```python
from build123d import *

# Parameters (mm, degrees)
PAD015_DEPTH        = 70.75
REVOLUTION002_ANGLE = 180
SKETCH027_R         = 1.375
POCKET008_DEPTH     = 17.751
SKETCH028_R         = 2.5
POCKET009_DEPTH     = 9.751
FILLET001_R         = 0.75


with BuildPart() as part:
    # Sketch025 → Pad015 (new body)
    with BuildSketch(Plane.XZ):
        with BuildLine():
            ThreePointArc((-11.975, 0), (0, -11.975), (11.975, 0))
            Line((11.975, 0), (17.754952, 0))
            Line((17.754952, -8), (17.754952, 0))
            Line((15.844952, -8), (17.754952, -8))
            ThreePointArc((-15.844952, -8), (0, -17.75), (15.844952, -8))
            Line((-15.844952, -8), (-17.754952, -8))
            Line((-17.754952, -8), (-17.754952, 0))
            Line((-17.754952, 0), (-11.975, 0))
        make_face()
    extrude(amount=PAD015_DEPTH)

    # Sketch026 (on Face3 of Pad015) → Revolution002 (revolve)
    with BuildSketch(Plane(origin=(0, 0, 0), x_dir=(-1, 0, 0), z_dir=(0, 0, 1))):
        Polygon((13.187436, 69.95), (11.975, 70.65), (10.762564, 69.95), (10.762564, 68.55), (11.975, 67.85), (13.187436, 68.55), align=None)
        Polygon((13.187436, 2.3), (11.975, 3), (10.762564, 2.3), (10.762564, 0.9), (11.975, 0.2), (13.187436, 0.9), align=None)
    revolve(axis=Axis((0, 0, 0), (0, -1, 0)), revolution_arc=REVOLUTION002_ANGLE)

    # Sketch027 (on Face18 of Revolution002) → Pocket008 (cut, through all)
    with BuildSketch(Plane(origin=(0, 0, 0), x_dir=(-1, 0, 0), z_dir=(0, 0, 1))):
        with Locations((-14.915, 63.75)):
            Circle(SKETCH027_R)
        with Locations((14.915, 63.75)):
            Circle(SKETCH027_R)
        with Locations((14.915, 7)):
            Circle(SKETCH027_R)
        with Locations((-14.915, 7)):
            Circle(SKETCH027_R)
    extrude(amount=-POCKET008_DEPTH, mode=Mode.SUBTRACT)

    # Sketch028 (on Face20 of Pocket008) → Pocket009 (cut, through all)
    with BuildSketch(Plane(origin=(0, 0, -8), x_dir=(1, 0, 0), z_dir=(0, 0, -1))):
        with Locations((-14.915, 63.75)):
            Circle(SKETCH028_R)
        with Locations((14.915, 63.75)):
            Circle(SKETCH028_R)
        with Locations((14.915, 7)):
            Circle(SKETCH028_R)
        with Locations((-14.915, 7)):
            Circle(SKETCH028_R)
    extrude(amount=POCKET009_DEPTH, mode=Mode.SUBTRACT)

    # Fillet001
    fillet001_edges = [part.edges().sort_by_distance(p)[0] for p in [
        (-17.754952, 0, -4),
        (-17.754952, -35.375, -8),
        (-16.799952, 0, -8),
        (0, 0, -17.75),
        (16.799952, 0, -8),
        (17.754952, 0, -4),
        (17.754952, -35.375, -8),
        (17.754952, -70.75, -4),
        (16.799952, -70.75, -8),
        (0, -70.75, -17.75),
        (-16.799952, -70.75, -8),
    ]]
    fillet(fillet001_edges, radius=FILLET001_R)


solid = part.part
```
Source: CAD feature listing. Evaluate the final solid. Frame: model axes, mm. A direction names the side the tool comes from. Give positions to 0.01 mm unless a question says otherwise; leave off trailing zeros. Loops run counter-clockwise (first coordinate to the right, second up) from the corner with the lowest first, then second, coordinate; pieces in that order, holes last. Notation, with made-up numbers: (89, -18.75) -> (145, -18.75) arc R27 ccw to (145, -1.75) -> close; hole circle Ø4 at (14, -17). An arc over 180 degrees is marked (long way). Use a Markdown table: item, result. Add a question column.
(1) First-contact query: pin 1 Ø4.5 at (x, y) = (-14.915, -63.75) entering from +Z; pin 2 Ø2.5 at (x, y) = (-15, -40.5) entering from -Z (3 decimals); pin 3 Ø8 at (x, y) = (14.915, -63.75) entering from -Z; pin 4 Ø5 at (x, y) = (14.5, -41) entering from -Z. Flat tips, straight axial feed; report the tip coordinate or a pass-through.
(2) Section query D-D (z = -1.75). Count the separate pieces of the cut face and the enclosed holes in it, then the cut area to 3 significant figures.
(3) Section query A-A (y = -63.75). Output: boundary loops of the cut face in (x, z) (3 decimals).
(4) Pull-direction query (Y, two-part tool) for faces 3 (the face through (-0.24, -1.59, -10.76)), 4 (the face through (16, -38, -8)), 5 (the face through (-0.24, -70.06, -10.95)); classes: +Y half, -Y half, draft (parallel to the pull), parting line (faces both ways), or undercut.
(5) Ray query, line 1 (X direction, y = -7, z = -3); line 2 (X direction, y = -63.75, z = -3.5); line 3 (Z direction, x = 16, y = -47). Return the intervals inside material, ascending.
(6) Access query for faces 1 (the face through (15.213, -62.408, -3.944)), 2 (the face through (-0.24, -68.43, -10.97)). Directions: +Z, -Z, +X, -X, +Y, -Y. A direction counts if a zero-diameter tool reaches every point of the face in a straight line with its end or side. Return the directions, or none.
(7) Section query C-C (y = -29). Output: boundary loops of the cut face in (x, z) (3 decimals).
(8) Section query B-B (x = 0). Output: boundary loops of the cut face in (y, z) (3 decimals).
Checked values:
| question | item | result |
|---|---|---|
| 1 | pin 1 | z = 0 |
| 1 | pin 2 | z = -11.225 |
| 1 | pin 3 | z = -14 |
| 1 | pin 4 | z = -13.08 |
| 2 | separate pieces | 2 |
| 2 | enclosed holes | 4 |
| 2 | area | 822 mm^2 |
| 3 | outline | (-17.755, -7.25) arc R0.75 ccw to (-17.005, -8) -> (-16.29, -8) -> (-16.29, 0) -> (-17.755, 0) -> close; (-13.54, -8) -> (-12.415, -8) -> (-12.415, -12.686) arc R17.75 ccw to (12.415, -12.686) -> (12.415, -8) -> (13.54, -8) -> (13.54, 0) -> (11.975, 0) arc R11.975 cw to (-11.975, 0) -> (-13.54, 0) -> close; (16.29, -8) -> (17.005, -8) arc R0.75 ccw to (17.755, -7.25) -> (17.755, 0) -> (16.29, 0) -> close |
| 4 | face 3 | draft |
| 4 | face 4 | undercut |
| 4 | face 5 | -Y half |
| 5 | line 1 | -17.75 to -16.29, -13.54 to -11.59, 11.59 to 13.54, 16.29 to 17.75 |
| 5 | line 2 | -17.75 to -16.29, -13.54 to -11.45, 11.45 to 13.54, 16.29 to 17.75 |
| 5 | line 3 | -8 to 0 |
| 6 | face 1 | +Z, -Z |
| 6 | face 2 | +Z |
| 7 | outline | (-17.755, -7.25) arc R0.75 ccw to (-17.005, -8) -> (-15.845, -8) arc R17.75 ccw to (15.845, -8) -> (17.005, -8) arc R0.75 ccw to (17.755, -7.25) -> (17.755, 0) -> (11.975, 0) arc R11.975 cw to (-11.975, 0) -> (-17.755, 0) -> close |
| 8 | outline | (-70.75, -17) arc R0.75 ccw to (-70, -17.75) -> (-0.75, -17.75) arc R0.75 ccw to (0, -17) -> (0, -11.975) -> (-0.2, -11.975) -> (-0.9, -10.763) -> (-2.3, -10.763) -> (-3, -11.975) -> (-67.85, -11.975) -> (-68.55, -10.763) -> (-69.95, -10.763) -> (-70.65, -11.975) -> (-70.75, -11.975) -> close |
